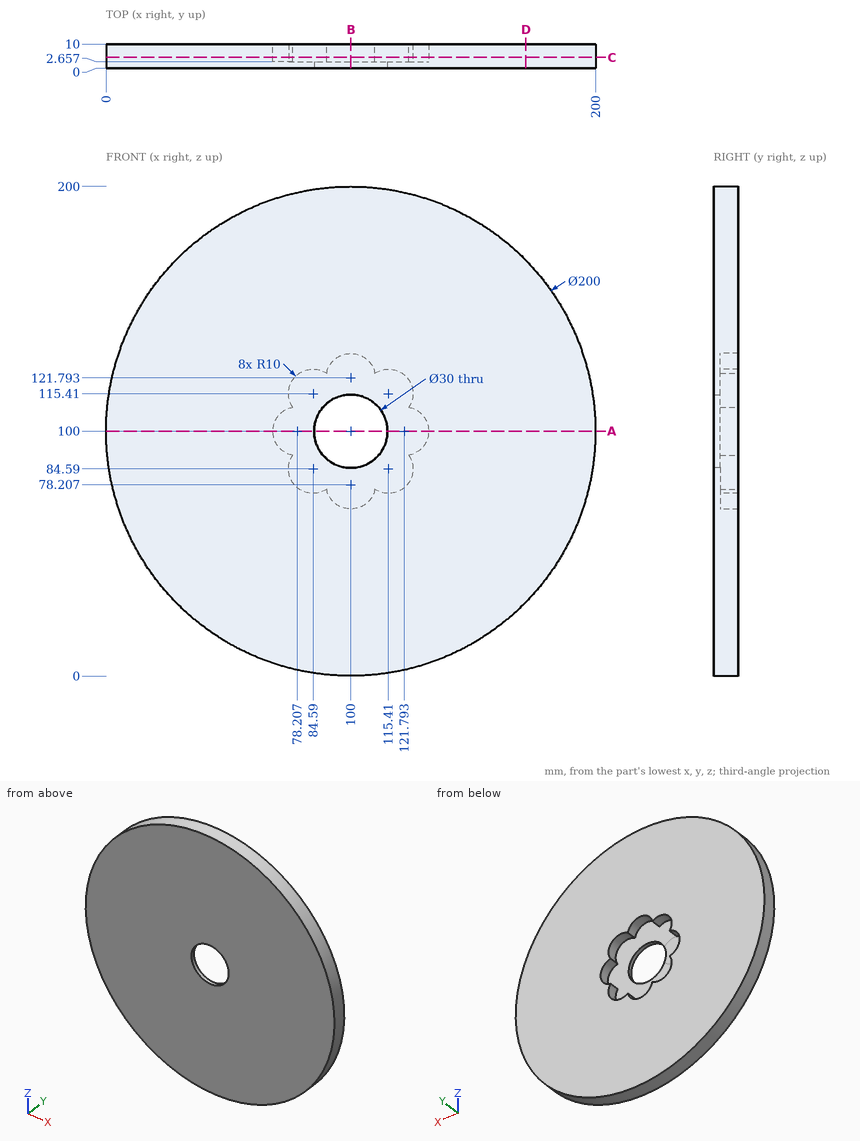
Can you work these out from the drawing? Everything is in mm from the part's minimum corner. Round coordinates to 2 decimals unless told otherwise and drop trailing zeros. Write each loop counter-clockwise with the first axis right and the second up, starting at its lowest first coordinate (ties: lowest second). Pieces come first, ordered by that corner, then holes.
1. I need wall thicknesses on L1, parallel to X at y = 1.8, z = 100; L2, parallel to X at y = 6.5, z = 99.5; L3, parallel to Y at x = 82, z = 110. Which ranges of each line are inside material? Lowest first, please.
2. Suppose I cut it at D-D (x = 171.5). List the corners of the cut face in (y, z) for me, and give its area (3 significant figures).
3. Suppose I cut it at B-B (x = 100). List the corners of the cut face in (y, z) for me, and give its area (3 significant figures).
4. Will these pins go through, and if not, where does the flat tip stop? pin 1 Ø18 at (x, z) = (100, 100) entering from +Y; pin 2 Ø14.5 at (x, z) = (76.5, 98) entering from +Y; pin 3 Ø4 at (y, z) = (7.5, 170) entering from -X; pin 4 Ø1.5 at (x, y) = (69, 8.5) entering from -Z (1 decimal).
5. Suppose I cut it at A-A (z = 100). List the corners of the cut face in (x, y) for me.
6. Suppose I cut it at C-C (y = 4.5). List the corners of the cut face in (x, z) for me.
Answer sheet:
1. L1: x = 0 to 85, 115 to 200
1. L2: x = 0 to 68.22, 131.78 to 200
1. L3: y = 0 to 2.66
2. outline: (0, 30.09) - (10, 30.09) - (10, 169.91) - (0, 169.91) - close
2. area: 1,400 mm2
3. outline: (0, 0) - (10, 0) - (10, 68.21) - (2.66, 68.21) - (2.66, 85) - (0, 85) - close; (0, 115) - (2.66, 115) - (2.66, 131.79) - (10, 131.79) - (10, 200) - (0, 200) - close
3. area: 1,450 mm2
4. pin 1: passes through
4. pin 2: stops at y = 2.66
4. pin 3: stops at x = 26.68
4. pin 4: stops at z = 4.7
5. outline: (0, 0) - (85, 0) - (85, 2.66) - (68.21, 2.66) - (68.21, 10) - (0, 10) - close; (115, 0) - (200, 0) - (200, 10) - (131.79, 10) - (131.79, 2.66) - (115, 2.66) - close
6. outline: circle Ø200 at (100, 100); hole (76.3, 90.18) arc R10 ccw to (90.18, 76.3) arc R10 ccw to (109.82, 76.3) arc R10 ccw to (123.7, 90.18) arc R10 ccw to (123.7, 109.82) arc R10 ccw to (109.82, 123.7) arc R10 ccw to (90.18, 123.7) arc R10 ccw to (76.3, 109.82) arc R10 ccw to start
